The model under review builds one solid part; all positions refer to its coordinate system, in mm. A direction names the side the tool comes from. Coordinates: 2 decimals unless noted, no trailing zeros. Write each loop counter-clockwise with the first axis right and the second up, starting at its lowest first coordinate (ties: lowest second). Pieces come first, ordered by that corner, then holes. Notation, with made-up numbers: (31.25, 67.25) - (78.25, 67.25) arc R27 cw to (78.25, 90.25) - close; hole circle Ø4 at (83.25, 8). An arc over 180 degrees is marked (long way). Put each result on its own line as item: value.
from build123d import *

# Parameters (mm, degrees)
SKETCH2_R                        = 9.525
SKETCH2_R_2                      = 5
BOSS_EXTRUDE1_DEPTH              = 19.05
SKETCH2_3_R                      = 5
BOSS_EXTRUDE2_DEPTH              = 19.05
F_11_32_0_34375_DIAMETER_HOLE1_D = 8.73125
SKETCH13_R                       = 8.509
CUT_EXTRUDE1_DEPTH               = 17.78


with BuildPart() as part:
    # Sketch2 → Boss-Extrude1 (new body)
    # profile 1 of 2: a face of its own
    with BuildSketch(Plane(origin=(0, 0, 0), x_dir=(1, 0, 0), z_dir=(0, 1, 0))):
        with Locations(Location((0, 0, 0), (0, 0, 90))):
            Circle(SKETCH2_R)
        Circle(SKETCH2_R_2, mode=Mode.SUBTRACT)
    # profile 2 of 2: a face of its own
    with BuildSketch(Plane(origin=(0, 0, 0), x_dir=(1, 0, 0), z_dir=(0, 1, 0))):
        Circle(SKETCH2_R_2)
    extrude(amount=BOSS_EXTRUDE1_DEPTH)

    # Sketch2<3> → Boss-Extrude2 (add)
    with BuildSketch(Plane(origin=(0, 0, 0), x_dir=(1, 0, 0), z_dir=(0, 1, 0))):
        with Locations(Location((0, 0, 0), (0, 0, 270))):
            Circle(SKETCH2_3_R)
    extrude(amount=-BOSS_EXTRUDE2_DEPTH)

    # 11/32 (0.34375) Diameter Hole1 (through all)
    with Locations(Plane(origin=(0, -19.05, 0), x_dir=(-1, 0, 0), z_dir=(0, -1, 0))):
        with Locations((0, 0)):
            Hole(F_11_32_0_34375_DIAMETER_HOLE1_D / 2)

    # Sketch13 → Cut-Extrude1 (cut)
    with BuildSketch(Plane(origin=(0, 19.05, 0), x_dir=(1, 0, 0), z_dir=(0, 1, 0))):
        with Locations(Location((0, 0, 0), (0, 0, 270))):
            Circle(SKETCH13_R)
    extrude(amount=-CUT_EXTRUDE1_DEPTH, mode=Mode.SUBTRACT)


solid = part.part
1. Machinability: for faces 4 (the flat face through (-4, 1.27, 4)), 5 (the cylindrical face through (5.796, 9.392, 7.559)), which of the approach directions +Z, -Z, +X, -X, +Y, -Y give a long, thin tool a straight path to every point of the face, cutting with its end or side? Answer none if there is none.
Determined:
face 4: +Y
face 5: +Y, -Y
2. Consider section C-C on y = -8.5. State the section outline as (x, z) points.
Determined:
outline: circle Ø10 at (0, 0); hole circle Ø8.73 at (0, 0)
3. Consider section B-B on x = 0. State the section outline as (y, z) points (3 decimals).
Determined:
outline: (-19.05, -5) - (0, -5) - (0, -9.525) - (19.05, -9.525) - (19.05, -8.509) - (1.27, -8.509) - (1.27, -4.366) - (-19.05, -4.366) - close; (-19.05, 4.366) - (1.27, 4.366) - (1.27, 8.509) - (19.05, 8.509) - (19.05, 9.525) - (0, 9.525) - (0, 5) - (-19.05, 5) - close
4. The part is to be moulded in two halves that separate along Z. For faces 1 (the cylindrical face through (-4.88, -9.39, -1.08)), 2 (the cylindrical face through (8.437, 10.284, -1.108)), 3 (the flat face through (4, 0, 4)), say which applies: +Z half, -Z half, draft (parallel to the pull), parting line (faces both ways), or undercut.
Determined:
face 1: parting line
face 2: undercut
face 3: draft
5. Consider section D-D on z = 7. State the section outline as (x, y) points, plus the area to 3 significant figures.
Determined:
outline: (-6.46, 0) - (6.46, 0) - (6.46, 19.05) - (4.84, 19.05) - (4.84, 1.27) - (-4.84, 1.27) - (-4.84, 19.05) - (-6.46, 19.05) - close
area: 74.1 mm^2
6. For pin 1 Ø2 at (x, y) = (5, -12) entering from -Z; pin 2 Ø5 at (x, z) = (2.5, -5.5) entering from -Y; pin 3 Ø7 at (x, z) = (0, 0) entering from +Y (1 decimal); pin 4 Ø4 at (y, z) = (-14.5, 4) entering from +X, all flat-tipped, find the tip position at first contact; note any pin that passes through.
Determined:
pin 1: stops at z = -3
pin 2: stops at y = -19.05
pin 3: passes through
pin 4: stops at x = 4.58
7. To check wall thickness, follow probe 1 along X at (y, z) = (5.5, 0) (3 decimals); probe 2 along X at (y, z) = (7, -5); probe 3 along Y at (x, z) = (8.75, -0.75). State the ranges of each line that lie inside material, in increasing order.
Determined:
probe 1: x = -9.525 to -8.509, 8.509 to 9.525
probe 2: x = -8.11 to -6.88, 6.88 to 8.11
probe 3: y = 0 to 19.05
8. Consider section A-A on z = 0. State the section outline as (x, y) points (3 decimals), plus the area to 3 significant figures.
Determined:
outline: (-9.525, 0) - (-5, 0) - (-5, -19.05) - (-4.366, -19.05) - (-4.366, 1.27) - (-8.509, 1.27) - (-8.509, 19.05) - (-9.525, 19.05) - close; (4.366, -19.05) - (5, -19.05) - (5, 0) - (9.525, 0) - (9.525, 19.05) - (8.509, 19.05) - (8.509, 1.27) - (4.366, 1.27) - close
area: 73.4 mm^2
